Design review of the part built by this model. Coordinates are the model's own, in mm. Give positions to 0.01 mm unless a question says otherwise; leave off trailing zeros. Write each loop counter-clockwise with the first axis right and the second up, starting at its lowest first coordinate (ties: lowest second). Pieces come first, ordered by that corner, then holes.
Autodesk Inventor part; units mm, degrees
ref_plane "YZ Plane" through (0, 0, 0) normal (1, 0, 0) x (0, 1, 0)
ref_plane "XZ Plane" through (0, 0, 0) normal (0, 1, 0) x (-1, 0, 0)
ref_plane "XY Plane" through (0, 0, 0) normal (0, 0, 1) x (1, 0, 0)
sketch "Boceto1" plane through (0, 0, 0) normal (0, 1, 0) x (-1, 0, 0)
  circle A0 centre (0, 0) radius 5
  line L0 (9.66, 9.91) -> (-30.22, 9.91)
  line L1 (-30.22, 9.91) -> (-30.22, -9.91)
  line L2 (-30.22, -9.91) -> (9.66, -9.91)
  line L3 (9.66, -9.91) -> (9.66, 9.91)
  circle A1 centre (-33.79, 5.085) radius 2
  circle A2 centre (13.47, -5.085) radius 2
  circle A3 centre (13.47, 5.085) radius 2
  circle A4 centre (-33.79, -5.085) radius 2
  line L4 (20, 15) -> (-40, 15)
  line L5 (-40, 15) -> (-40, -15)
  line L6 (-40, -15) -> (20, -15)
  line L7 (20, -15) -> (20, 15)
  line L8 (20, -15) -> (10, -15)
  line L9 (10, -15) -> (10, -25)
  line L10 (10, -25) -> (20, -25)
  line L11 (20, -25) -> (20, -15)
  line L12 (20, 15) -> (10, 15)
  line L13 (10, 15) -> (10, 25)
  line L14 (10, 25) -> (20, 25)
  line L15 (20, 25) -> (20, 15)
  circle A5 centre (15, 20) radius 2
  circle A6 centre (15, -20) radius 2
  line L16 (-10, -15) -> (-40, -15)
  line L17 (-40, -15) -> (-40, -18.18)
  line L18 (-40, -18.18) -> (-10, -18.18)
  line L19 (-10, -18.18) -> (-10, -15)
  line L20 (-10, 18.18) -> (-40, 18.18)
  line L21 (-40, 18.18) -> (-40, 15)
  line L22 (-40, 15) -> (-10, 15)
  line L23 (-10, 15) -> (-10, 18.18)
  dimension "d0" = 10
  dimension "d1" = 9.91
  dimension "d2" = 19.82
  dimension "d3" = 9.66
  dimension "d4" = 39.88
  dimension "d5" = 4
  dimension "d6" = 4
  dimension "d7" = 4
  dimension "d8" = 5.085
  dimension "d9" = 10.17
  dimension "d10" = 13.47
  dimension "d11" = 13.47
  dimension "d12" = 4
  dimension "d13" = 33.79
  dimension "d14" = 33.79
  dimension "d15" = 5.085
  dimension "d16" = 10.17
  dimension "d25" = 15
  dimension "d26" = 30
  dimension "d27" = 60
  dimension "d28" = 40
  dimension "d29" = 10
  dimension "d30" = 10
  dimension "d31" = 10
  dimension "d32" = 4
  dimension "d33" = 4
  dimension "d34" = 5
  dimension "d35" = 5
  dimension "d36" = 5
  dimension "d37" = 5
  dimension "d38" = 3.18
  dimension "d39" = 30
extrude "Extrusión1" add sketch "Boceto1" along normal blind 1 contours L7 L6 L5 L4 | L4 L13 L14 L15 | L11 L10 L9 L6 | L4 L21 L20 L23 | L19 L18 L17 L6
properties part number "PINZA_SOST.SERVO"
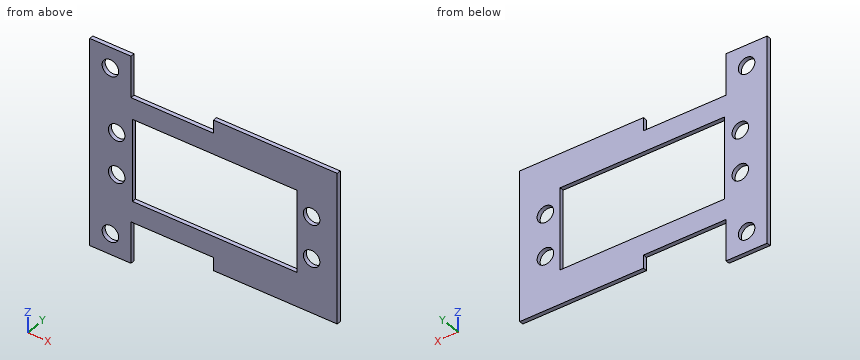
(1) To check wall thickness, follow L1, parallel to Z at x = 33.79, y = 0.55 (3 decimals); L2, parallel to X at y = 0.6, z = 5; L3, parallel to X at y = 0.1, z = -17. State the ranges of each line that lie inside material, in increasing order.
Resolved:
L1: z = -18.18 to -7.085, -3.085 to 3.085, 7.085 to 18.18
L2: x = -20 to -15.47, -11.47 to -9.66, 30.22 to 31.79, 35.79 to 40
L3: x = -20 to -10, 10 to 40
(2) Clearance check with flat-ended pins moving along their axes: P1, Ø5, axis at x = -15, z = -20, coming from the +Y side; P2, Ø0.5, axis at x = -3, y = 0.5, coming from the +Z side; P3, Ø1, axis at x = -1.5, z = -16, coming from the +Y side; P4, Ø0.5, axis at y = 0.5, z = 18.5, coming from the +X side. State where each tip first meets the part, or that it passes through.
Resolved:
P1: stops at y = 1
P2: stops at z = 15
P3: passes through
P4: stops at x = -10
(3) Consider section C-C, the plane z = 9. Give the boundary of the cut face in (x, y), then the cut area to 3 significant figures.
Resolved:
outline: (-20, 0) - (-9.66, 0) - (-9.66, 1) - (-20, 1) - close; (30.22, 0) - (40, 0) - (40, 1) - (30.22, 1) - close
area: 20.1 mm2
(4) Consider section A-A, the plane x = 33.79. Give the boundary of the cut face in (y, z) (3 decimals).
Resolved:
outline: (0, -18.18) - (1, -18.18) - (1, -7.085) - (0, -7.085) - close; (0, -3.085) - (1, -3.085) - (1, 3.085) - (0, 3.085) - close; (0, 7.085) - (1, 7.085) - (1, 18.18) - (0, 18.18) - close
(5) Consider section B-B, the plane x = -8.5. Give the boundary of the cut face in (y, z), then the cut area to 3 significant figures.
Resolved:
outline: (0, -15) - (1, -15) - (1, -9.91) - (0, -9.91) - close; (0, 9.91) - (1, 9.91) - (1, 15) - (0, 15) - close
area: 10.2 mm2
